Source: three-view drawing plus pictorial views. Frame: mm from the lowest corner of the part. Round coordinates to 2 decimals unless told otherwise and drop trailing zeros. Order: outer loops, then holes, each group sorted by start corner. A loop starts at its lowest first (then second) coordinate and runs counter-clockwise, first axis right, second up. Notation, with made-up numbers: (35.5, -13.5) -> (51.5, -13.5) arc R21 cw to (51.5, 13.5) -> close; hole circle Ø3 at (83.5, 54.5). An arc over 180 degrees is marked (long way). Answer as CSV lines item,"result". Start each with the question number.
1) Section query B-B, the plane z = 252. Output: boundary loops of the cut face in (x, y).
2) Section query A-A, the plane y = 4.25. Output: boundary loops of the cut face in (x, z) (3 decimals), and give its area (3 significant figures).
3) Line query: L1, parallel to Z at x = 300.5, y = 9 (3 decimals); L2, parallel to X at y = 6, z = 249; L3, parallel to X at y = 7, z = 116.5. Output: solid intervals per line, ascending.
4) First-contact query: P1, Ø9.5, axis at x = 5.5, y = 11, coming from the +Z side (3 decimals); P2, Ø1, axis at x = 372, z = 382.5, coming from the -Y side; P3, Ø1.5, axis at y = 9, z = 253.5, coming from the +X side; P4, Ø4, axis at x = 235.5, z = 418, coming from the -Y side (3 decimals). Flat tips, straight axial feed; report the tip coordinate or a pass-through.
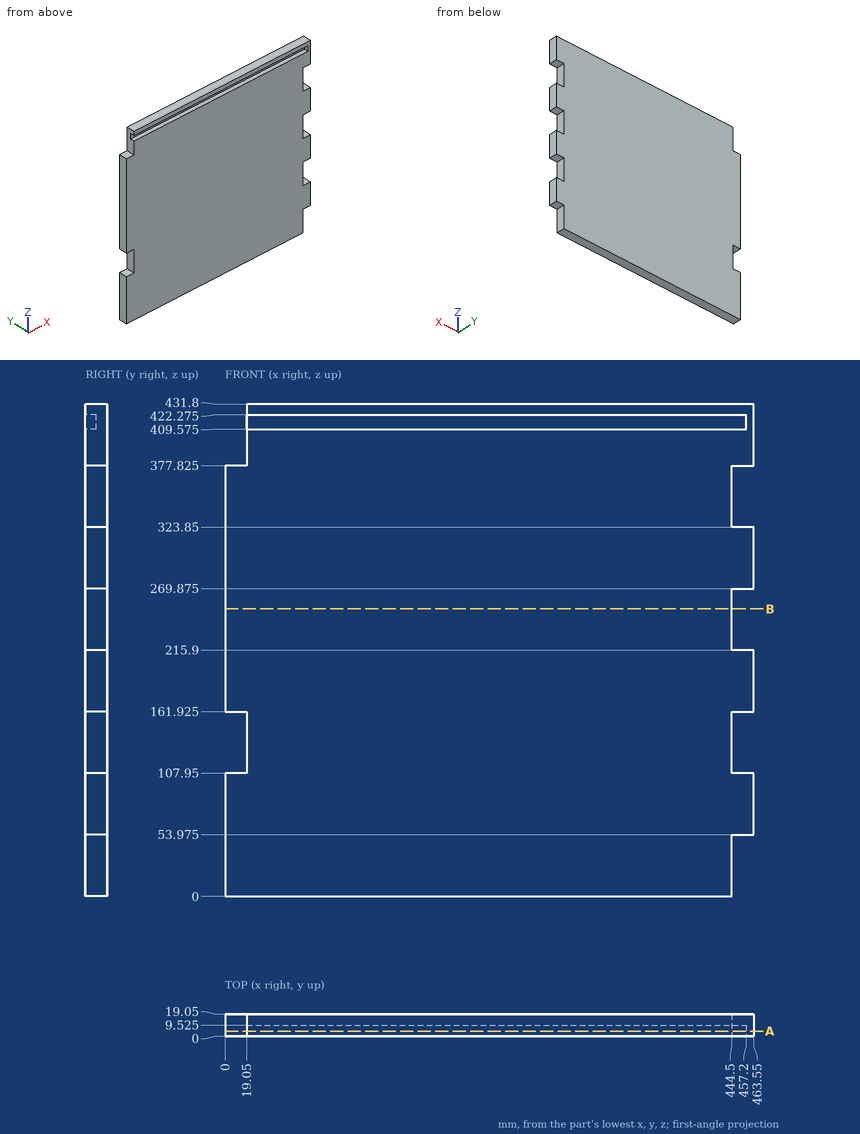
Findings:
1,outline,"(0, 0) -> (444.5, 0) -> (444.5, 19.05) -> (0, 19.05) -> close"
2,outline,"(0, 0) -> (444.5, 0) -> (444.5, 53.975) -> (463.55, 53.975) -> (463.55, 107.95) -> (444.5, 107.95) -> (444.5, 161.925) -> (463.55, 161.925) -> (463.55, 215.9) -> (444.5, 215.9) -> (444.5, 269.875) -> (463.55, 269.875) -> (463.55, 323.85) -> (444.5, 323.85) -> (444.5, 377.825) -> (463.55, 377.825) -> (463.55, 431.8) -> (19.05, 431.8) -> (19.05, 422.275) -> (457.2, 422.275) -> (457.2, 409.575) -> (19.05, 409.575) -> (19.05, 377.825) -> (0, 377.825) -> (0, 161.925) -> (19.05, 161.925) -> (19.05, 107.95) -> (0, 107.95) -> close"
2,area,"188,000 mm^2"
3,L1,"z = 0 to 409.575, 422.275 to 431.8"
3,L2,"x = 0 to 444.5"
3,L3,"x = 19.05 to 444.5"
4,P1,"stops at z = 377.825"
4,P2,"stops at y = 0"
4,P3,"stops at x = 444.5"
4,P4,"stops at y = 9.525"
